Verification items for the finished model (mm, model axes). Give positions to 0.01 mm unless a question says otherwise; leave off trailing zeros. Order: outer loops, then holes, each group sorted by start corner. A loop starts at its lowest first (then second) coordinate and runs counter-clockwise, first axis right, second up.
from build123d import *

# Parameters (mm, degrees)
SKETCH1_W                 = 150
SKETCH1_H                 = 150
BOSS_EXTRUDE1_DEPTH       = 3.18
SKETCH9_W                 = 3.18
SKETCH9_H                 = 9.9
SKETCH9_H_2               = 25.8
CUT_EXTRUDE7_DEPTH        = 10
MIRROR2_COPY_1_SKETCH_W   = 3.18
MIRROR2_COPY_1_SKETCH_H   = 9.9
MIRROR2_COPY_1_SKETCH_H_2 = 25.8
MIRROR2_COPY_1_DEPTH      = 10
SKETCH10_W                = 6.72
SKETCH10_H                = 3.18
SKETCH10_W_2              = 25.8
CUT_EXTRUDE8_DEPTH        = 10
MIRROR5_COPY_1_SKETCH_W   = 6.72
MIRROR5_COPY_1_SKETCH_H   = 3.18
MIRROR5_COPY_1_SKETCH_W_2 = 25.8
MIRROR5_COPY_1_DEPTH      = 10
SKETCH11_R                = 1.6
CUT_EXTRUDE9_DEPTH        = 10
SKETCH12_R                = 1.6
CUT_EXTRUDE10_DEPTH       = 10
SKETCH13_R                = 1.6
CUT_EXTRUDE11_DEPTH       = 10
SKETCH14_R                = 1.6
CUT_EXTRUDE12_DEPTH       = 10


with BuildPart() as part:
    # Sketch1 → Boss-Extrude1 (new body)
    with BuildSketch(Plane(origin=(0, 0, 0), x_dir=(1, 0, 0), z_dir=(0, 1, 0))):
        Rectangle(SKETCH1_W, SKETCH1_H)
    extrude(amount=BOSS_EXTRUDE1_DEPTH)

    # Sketch9 → Cut-Extrude7 (cut)
    with BuildSketch(Plane.XZ):
        with Locations((73.41, 70.05)):
            Rectangle(SKETCH9_W, SKETCH9_H)
        with Locations((73.41, 26)):
            Rectangle(SKETCH9_W, SKETCH9_H_2)
    cut_extrude7 = extrude(amount=-CUT_EXTRUDE7_DEPTH, mode=Mode.SUBTRACT)

    # Mirror1: Cut-Extrude7 across plane
    add(cut_extrude7.mirror(Plane.XY), mode=Mode.SUBTRACT)

    # Mirror2: Cut-Extrude7 across plane
    add(cut_extrude7.mirror(Plane(origin=(0, 0, 0), x_dir=(0, 0, 1), z_dir=(1, 0, 0))), mode=Mode.SUBTRACT)

    # Mirror2 copy 1 sketch → Mirror2 copy 1 (cut)
    with BuildSketch(Plane(origin=(0, 0, 0), x_dir=(-1, 0, 0), z_dir=(0, -1, 0))):
        with Locations((73.41, 70.05)):
            Rectangle(MIRROR2_COPY_1_SKETCH_W, MIRROR2_COPY_1_SKETCH_H)
        with Locations((73.41, 26)):
            Rectangle(MIRROR2_COPY_1_SKETCH_W, MIRROR2_COPY_1_SKETCH_H_2)
    extrude(amount=-MIRROR2_COPY_1_DEPTH, mode=Mode.SUBTRACT)

    # Sketch10 → Cut-Extrude8 (cut)
    with BuildSketch(Plane.XZ):
        with Locations((68.46, 73.41)):
            Rectangle(SKETCH10_W, SKETCH10_H)
        with Locations((26, 73.41)):
            Rectangle(SKETCH10_W_2, SKETCH10_H)
    cut_extrude8 = extrude(amount=-CUT_EXTRUDE8_DEPTH, mode=Mode.SUBTRACT)

    # Mirror4: Cut-Extrude8 across plane
    add(cut_extrude8.mirror(Plane(origin=(0, 0, 0), x_dir=(0, 0, 1), z_dir=(1, 0, 0))), mode=Mode.SUBTRACT)

    # Mirror5: Cut-Extrude8 across plane
    add(cut_extrude8.mirror(Plane.XY), mode=Mode.SUBTRACT)

    # Mirror5 copy 1 sketch → Mirror5 copy 1 (cut)
    with BuildSketch(Plane(origin=(0, 0, 0), x_dir=(-1, 0, 0), z_dir=(0, -1, 0))):
        with Locations((68.46, 73.41)):
            Rectangle(MIRROR5_COPY_1_SKETCH_W, MIRROR5_COPY_1_SKETCH_H)
        with Locations((26, 73.41)):
            Rectangle(MIRROR5_COPY_1_SKETCH_W_2, MIRROR5_COPY_1_SKETCH_H)
    extrude(amount=-MIRROR5_COPY_1_DEPTH, mode=Mode.SUBTRACT)

    # Sketch11 → Cut-Extrude9 (cut)
    with BuildSketch(Plane.XZ):
        with Locations((27.35, 28.6)):
            Circle(SKETCH11_R)
    extrude(amount=-CUT_EXTRUDE9_DEPTH, mode=Mode.SUBTRACT)

    # Sketch12 → Cut-Extrude10 (cut)
    with BuildSketch(Plane.XZ):
        with Locations((-20.95, 28.6)):
            Circle(SKETCH12_R)
    extrude(amount=-CUT_EXTRUDE10_DEPTH, mode=Mode.SUBTRACT)

    # Sketch13 → Cut-Extrude11 (cut)
    with BuildSketch(Plane.XZ):
        with Locations((27.35, -22.2)):
            Circle(SKETCH13_R)
    extrude(amount=-CUT_EXTRUDE11_DEPTH, mode=Mode.SUBTRACT)

    # Sketch14 → Cut-Extrude12 (cut)
    with BuildSketch(Plane.XZ):
        with Locations((-0.55, -23.360495604)):
            Circle(SKETCH14_R)
    extrude(amount=-CUT_EXTRUDE12_DEPTH, mode=Mode.SUBTRACT)


solid = part.part
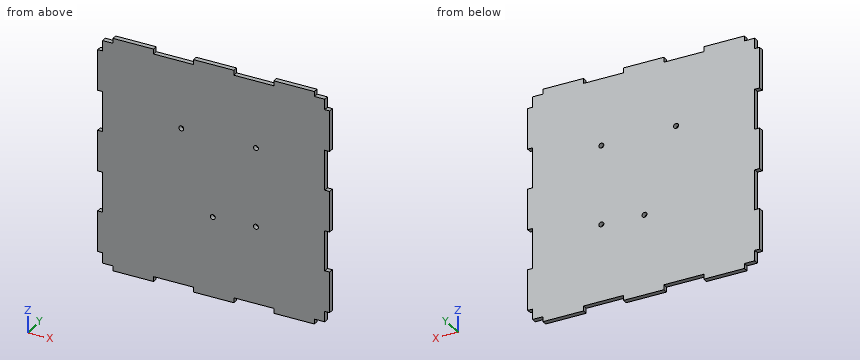
(1) Section check A-A, the plane y = 0.7. Give the number of separate pieces and of enclosed holes in the cut face, then the cut area to 3 significant figures.
Solved:
separate pieces: 1
enclosed holes: 4
area: 21,600 mm2
(2) Section check B-B, the plane x = 36.5. Enter the section's corners in (y, z), then the cut area to 3 significant figures.
Solved:
outline: (0, -71.82) - (3.18, -71.82) - (3.18, 71.82) - (0, 71.82) - close
area: 457 mm2
(3) Go/stop test with flat-tipped pins: pin 1 (1.6 mm diameter, centred on x = 73, y = 1, fed in from -Z); pin 2 (1.5 mm diameter, centred on y = 1.5, z = -18.5, fed in from +X); pin 3 (1.6 mm diameter, centred on x = -70, y = 1.5, fed in from +Z). Record where each tip stops, or that it passes through.
Solved:
pin 1: stops at z = -65.1
pin 2: stops at x = 71.82
pin 3: stops at z = 71.82
(4) Scan lines: line 1 (Z direction, x = 27.35, y = 2.35); line 2 (Z direction, x = -20.95, y = 1.3); line 3 (Z direction, x = -1, y = 0.5). Record each from-to range of solid material in increasing order.
Solved:
line 1: z = -71.82 to -23.8, -20.6 to 27, 30.2 to 71.82
line 2: z = -71.82 to 27, 30.2 to 71.82
line 3: z = -75 to -24.9, -21.83 to 75
(5) Section check C-C, the plane z = 19. Enter the section's corners in (x, y), then the cut area to 3 significant figures.
Solved:
outline: (-71.82, 0) - (71.82, 0) - (71.82, 3.18) - (-71.82, 3.18) - close
area: 457 mm2
